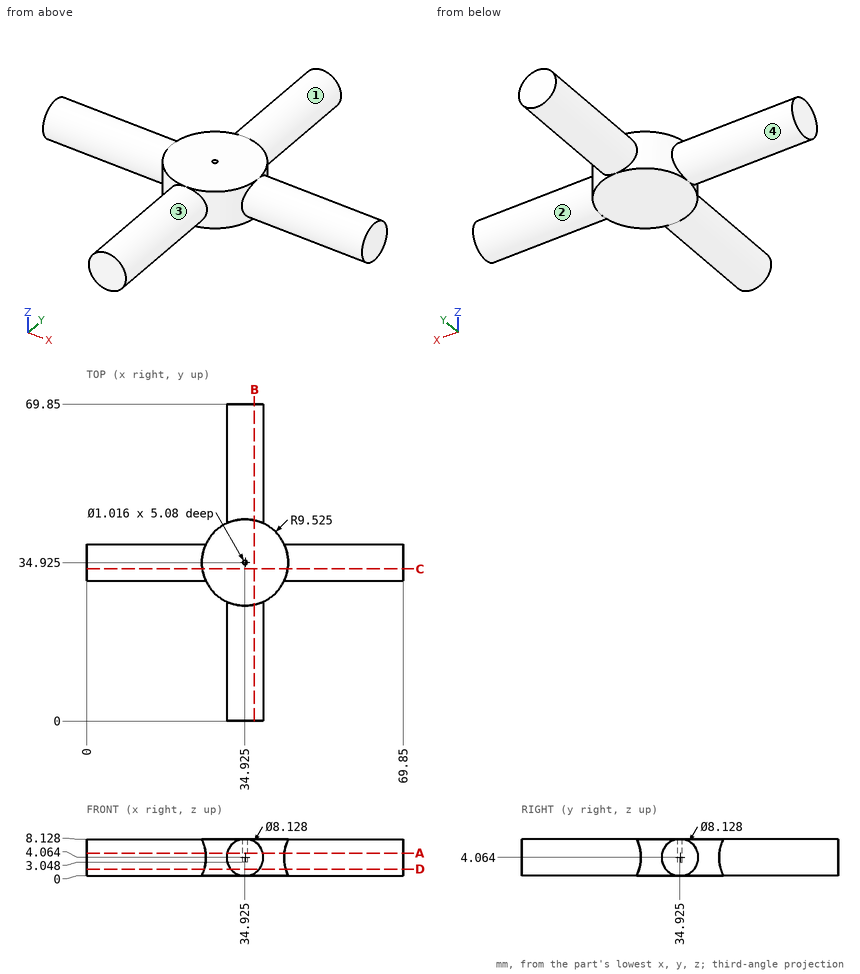
Job drawing, mm, ordinate dimensions from the low corner. One solid piece. A direction names the side the tool comes from. Give positions to 0.01 mm unless a question says otherwise; leave off trailing zeros. Order: outer loops, then holes, each group sorted by start corner. A loop starts at its lowest first (then second) coordinate and runs counter-clockwise, first axis right, second up. Notation, with made-up numbers: (76.5, 42.5) -> (81.5, 42.5) arc R23 ccw to (81.5, 74.5) -> close; hole circle Ø5 at (74.25, 60.5). An arc over 180 degrees is marked (long way). Return JSON: item names as keys, results as strings.
Q1. Saw through at B-B (x = 37). Write the cut outline in (y, z).
Working result:
{"outline": "(0, 0.57) -> (25.63, 0.57) -> (25.63, 0) -> (44.22, 0) -> (44.22, 0.57) -> (69.85, 0.57) -> (69.85, 7.56) -> (44.22, 7.56) -> (44.22, 8.13) -> (25.63, 8.13) -> (25.63, 7.56) -> (0, 7.56) -> close"}
Q2. Which spindle directions (+Z, -Z, +X, -X, +Y, -Y) get a long thin tool onto all of the face, cutting with end or side? Do the marked faces 1, 2, 3 and 4. Say none if no direction does.
Working result:
{"face 1": "+Y", "face 2": "+X", "face 3": "-Y", "face 4": "-X"}
Q3. Saw through at C-C (y = 33.5). Write the cut outline in (x, z).
Working result:
{"outline": "(0, 0.26) -> (25.51, 0.26) -> (25.51, 0) -> (44.34, 0) -> (44.34, 0.26) -> (69.85, 0.26) -> (69.85, 7.87) -> (44.34, 7.87) -> (44.34, 8.13) -> (25.51, 8.13) -> (25.51, 7.87) -> (0, 7.87) -> close"}
Q4. Drill centre lines: line 1 (X direction, y = 11, z = 4); line 2 (Y direction, x = 48, z = 3.75); line 3 (Y direction, x = 39, z = 3). Where is each one in solid material? Low to high.
Working result:
{"line 1": "30.86 to 38.99", "line 2": "30.87 to 38.98", "line 3": "26.32 to 43.53"}
Q5. Saw through at D-D (z = 1.5). Write the cut outline in (x, y) (3 decimals), then the cut area to 3 significant figures.
Working result:
{"outline": "(0, 31.772) -> (25.937, 31.772) arc R9.525 ccw to (31.772, 25.937) -> (31.772, 0) -> (38.078, 0) -> (38.078, 25.937) arc R9.525 ccw to (43.913, 31.772) -> (69.85, 31.772) -> (69.85, 38.078) -> (43.913, 38.078) arc R9.525 ccw to (38.078, 43.913) -> (38.078, 69.85) -> (31.772, 69.85) -> (31.772, 43.913) arc R9.525 ccw to (25.937, 38.078) -> (0, 38.078) -> close", "area": "930 mm²"}
Q6. Saw through at A-A (z = 5). Write the cut outline in (x, y) (3 decimals), then the cut area to 3 significant figures.
Working result:
{"outline": "(0, 30.97) -> (26.26, 30.97) arc R9.525 ccw to (30.97, 26.26) -> (30.97, 0) -> (38.88, 0) -> (38.88, 26.26) arc R9.525 ccw to (43.59, 30.97) -> (69.85, 30.97) -> (69.85, 38.88) -> (43.59, 38.88) arc R9.525 ccw to (38.88, 43.59) -> (38.88, 69.85) -> (30.97, 69.85) -> (30.97, 43.59) arc R9.525 ccw to (26.26, 38.88) -> (0, 38.88) -> close; hole circle Ø1.016 at (34.925, 34.925)", "area": "1,100 mm²"}
Q7. Flat gauge pins, fed straight in: pin 1 (0.8 mm diameter, centred on x = 34.925, y = 34.925, fed in from +Z); pin 2 (3 mm diameter, centred on x = 29, z = 1, fed in from -Y); pin 3 (3 mm diameter, centred on y = 42, z = 3.5, fed in from +X). Where does each tip first touch, or does it go through?
Working result:
{"pin 1": "z = 3.05", "pin 2": "y = 26.49", "pin 3": "x = 42.65"}
